Input: dimensioned drawing with shaded views. Units: mm. Origin: part minimum x, y, z. A direction names the side the tool comes from. Coordinates: 2 decimals unless noted, no trailing zeros. Order: outer loops, then holes, each group sorted by start corner. A loop starts at its lowest first (then second) coordinate and runs counter-clockwise, first axis right, second up. Notation, with made-up numbers: (2.25, 71) -> (25.25, 71) arc R22 cw to (25.25, 93) -> close; hole circle Ø11 at (-26, 36.25). An arc over 180 degrees is marked (long way). Write item = value, one per line. Start each with the question number.
Item 1: Mould query, pull axis Z, two halves, no side actions, for the marked faces 1, 2, 3 and 4. Classes: released by +Z, released by -Z, zero draft, split by the parting line, or undercut.
Item 2: Set-up query: the marked faces 5, 6, 7 and 8. Return all of +Z, -Z, +X, -X, +Y, -Y with unobstructed straight access to the full face (end or side cutting, diameter ignored); none if empty.
Item 3: Section query A-A (x = 4). Output: boundary loops of the cut face in (y, z), then the cut area to 3 significant figures.
Item 4: Section query B-B (z = 30). Output: boundary loops of the cut face in (x, y), then the cut area to 3 significant figures.
Item 5: Section query C-C (y = 3). Output: boundary loops of the cut face in (x, z).
Item 6: Contact query for flat-ended pins moving along their axis: pin 1 (10 mm diameter, centred on x = 42.5, z = 38, fed in from +Y); pin 2 (8 mm diameter, centred on y = 13, z = 29, fed in from +X); pin 3 (4 mm diameter, centred on y = 12, z = 40, fed in from +X). Output: stop coordinate, or through.
Item 7: Ray query, line 1 along X through (y, z) = (5, 30); line 2 along Z through (x, y) = (32, 14); line 3 along Y through (x, z) = (50, 13.5). Return the intervals inside material, ascending. Write a range as [from, to].
Item 8: Section query D-D (y = 9). Output: boundary loops of the cut face in (x, z), then the cut area to 3 significant figures.
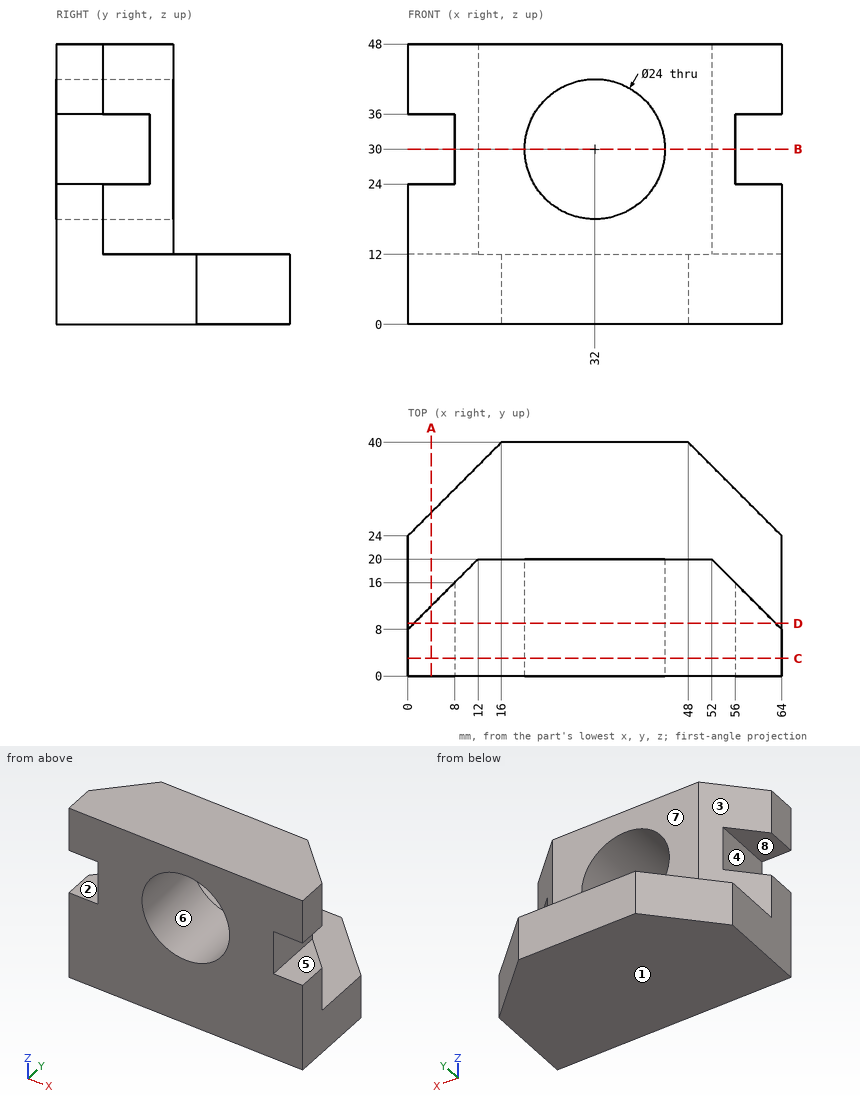
Computed:
q1.face_1 = released by -Z
q1.face_2 = undercut
q1.face_3 = zero draft
q1.face_4 = undercut
q2.face_5 = +X, +Y, -Y
q2.face_6 = +Y, -Y
q2.face_7 = +Z, +X, -X, +Y
q2.face_8 = -X, +Y, -Y
q3.outline = (0, 0) -> (28, 0) -> (28, 12) -> (12, 12) -> (12, 24) -> (0, 24) -> close; (0, 36) -> (12, 36) -> (12, 48) -> (0, 48) -> close
q3.area = 624 mm^2
q4.outline = (8, 0) -> (20, 0) -> (20, 20) -> (12, 20) -> (8, 16) -> close; (44, 0) -> (56, 0) -> (56, 16) -> (52, 20) -> (44, 20) -> close
q4.area = 464 mm^2
q5.outline = (0, 0) -> (64, 0) -> (64, 24) -> (56, 24) -> (56, 36) -> (64, 36) -> (64, 48) -> (0, 48) -> (0, 36) -> (8, 36) -> (8, 24) -> (0, 24) -> close; hole circle Ø24 at (32, 30)
q6.pin_1 = 20
q6.pin_2 = 56
q6.pin_3 = 62
q7.line_1 = [8, 20], [44, 56]
q7.line_2 = [0, 18], [42, 48]
q7.line_3 = [0, 20]
q8.outline = (0, 0) -> (64, 0) -> (64, 12) -> (63, 12) -> (63, 24) -> (56, 24) -> (56, 36) -> (63, 36) -> (63, 48) -> (1, 48) -> (1, 36) -> (8, 36) -> (8, 24) -> (1, 24) -> (1, 12) -> (0, 12) -> close; hole circle Ø24 at (32, 30)
q8.area = 2,380 mm^2
